Build history of the part. All positions in model axes, mm. Face numbers are marked on the shaded views. A direction names the side the tool comes from. Round coordinates to 2 decimals unless told otherwise and drop trailing zeros. Write each loop counter-clockwise with the first axis right and the second up, starting at its lowest first coordinate (ties: lowest second). Pieces come first, ordered by that corner, then holes. Notation, with made-up numbers: (60.5, 39.5) -> (81.5, 39.5) arc R25 ccw to (81.5, 66.5) -> close; hole circle Ø10 at (52, 14). An arc over 180 degrees is marked (long way). Return JSON: item names as keys, results as strings.
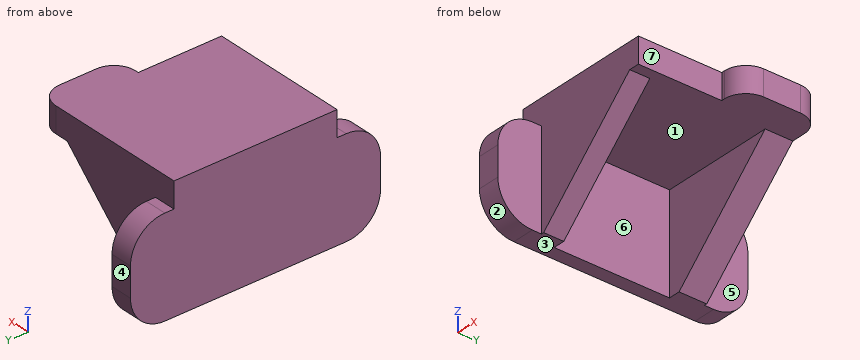
Autodesk Inventor part; units mm, degrees
ref_plane "YZ Plane" through (0, 0, 0) normal (1, 0, 0) x (0, 1, 0)
ref_plane "XZ Plane" through (0, 0, 0) normal (0, 1, 0) x (-1, 0, 0)
ref_plane "XY Plane" through (0, 0, 0) normal (0, 0, 1) x (1, 0, 0)
sketch "Sketch1" plane through (0, 0, 0) normal (0, 0, 1) x (1, 0, 0)
  line L0 (0, 0) -> (0, 60.76)
  line L1 (0, 60.76) -> (51.9, 60.76)
  line L2 (51.9, 31.06) -> (51.9, 0)
  line L3 (51.9, 0) -> (0, 0)
  line L4 (51.9, 60.76) -> (61.1, 60.76)
  line L5 (61.1, 60.76) -> (61.1, 31.06)
  line L6 (61.1, 31.06) -> (51.9, 31.06)
  dimension "d0" = 60.76
  dimension "d1" = 51.9
  dimension "d2" = 9.2
  dimension "d3" = 29.7
extrude "Extrusion1" add sketch "Sketch1" along normal blind 9.5
fillet "Fillet1" radius 8 2 edges at (61.1, 60.76, 4.75) (61.1, 31.06, 4.75)
sketch "Sketch2" plane through (0, 0, 0) normal (0, -1, 0) x (1, 0, 0)
  line L0 (51.9, 0) -> (0, 0)
  line L1 (0, -36.5) -> (0, 0)
  line L2 (0, -36.5) -> (9.3, -36.5)
  line L3 (9.3, -36.5) -> (48, 0)
  point P0 (0, 9.5)
  dimension "d7" = 46
  dimension "d8" = 3.9
  dimension "d9" = 9.3
extrude "Extrusion2" add sketch "Sketch2" against normal blind 7.5
sketch "Sketch3" plane through (0, 60.76, 9.5) normal (0, 1, 0) x (1, 0, 0)
  line L0 (0, 46) -> (0, 9.5)
  line L1 (48, 9.5) -> (0, 9.5)
  line L2 (48, 9.5) -> (9.3, 46)
  line L3 (9.3, 46) -> (0, 46)
extrude "Extrusion3" add sketch "Sketch3" against normal blind 10.3
sketch "Sketch4" plane through (0, 0, 9.5) normal (-1, 0, 0) x (0, 0, 1)
  line L0 (-46, 60.76) -> (0, 60.76)
  line L1 (-9.5, 7.5) -> (-9.5, 50.46)
  line L2 (-46, 0) -> (-46, 7.5)
  line L3 (-46, -16.2) -> (-46, 76.96)
  line L4 (-9.5, 76.96) -> (-9.5, -16.2)
  line L5 (-9.5, -16.2) -> (-46, -16.2)
  line L6 (-9.5, 76.96) -> (-46, 76.96)
  point P0 (-9.5, 0)
  dimension "d15" = 93.16
  dimension "d16" = 16.2
extrude "Extrusion4" add sketch "Sketch4" against normal blind 8.3
sketch "Sketch5" plane through (8.3, 0, 9.5) normal (1, 0, 0) x (0, 0, -1)
  line L0 (9.5, 50.46) -> (46, 50.46)
  line L1 (9.5, 7.5) -> (9.5, 50.46)
  line L2 (46, 7.5) -> (9.5, 7.5)
  line L3 (46, 7.5) -> (46, 50.46)
  point P0 (9.5, 0)
extrude "Extrusion5" cut sketch "Sketch5" against normal blind 3.3
fillet "Fillet2" radius 12.8 4 edges at (4.15, 76.96, -36.5) (4.15, -16.2, -36.5) (4.15, -16.2, 0) (4.15, 76.96, 0)
properties part number "FelixOriginalBase"
Q1. Saw through at D-D on y = 27.5. List the corners of the cut face in (x, z).
Verdict:
{"outline": "(0, -36.5) -> (5, -36.5) -> (5, 0) -> (51.9, 0) -> (51.9, 9.5) -> (0, 9.5) -> close"}
Q2. Pin check, flat tips, straight feed: pin 1 Ø1.7 at (x, y) = (6, 62) entering from +Z; pin 2 Ø5 at (x, z) = (42.5, -3) entering from -Y; pin 3 Ø8 at (x, z) = (34.5, 4) entering from +Y. Stop position of each tip, or through.
Verdict:
{"pin 1": "stops at z = 0", "pin 2": "stops at y = 0", "pin 3": "stops at y = 60.76"}
Q3. 3-axis set-ups, long thin cutter, end or side, ignore diameter. For the marked faces 4, 5, 6 and 7: which of +Z, -Z, +X, -X, +Y, -Y reach the whole face in a straight line?
Verdict:
{"face 4": "+Z, -Z, +X, -X, +Y", "face 5": "+Z, -Z, +X, +Y", "face 6": "-Z, +X", "face 7": "+Z, -Z, +X, -Y"}
Q4. Saw through at A-A on y = 6.5. List the corners of the cut face in (x, z), then the cut area to 3 significant figures.
Verdict:
{"outline": "(0, -36.5) -> (9.3, -36.5) -> (48, 0) -> (51.9, 0) -> (51.9, 9.5) -> (0, 9.5) -> close", "area": "1,540 mm²"}
Q5. Saw through at B-B on x = 36.5. List the corners of the cut face in (y, z), then the cut area to 3 significant figures.
Verdict:
{"outline": "(0, -10.85) -> (7.5, -10.85) -> (7.5, 0) -> (50.46, 0) -> (50.46, -10.85) -> (60.76, -10.85) -> (60.76, 9.5) -> (0, 9.5) -> close", "area": "770 mm²"}
Q6. Two-plate mould, pull along Y, no slides. Class the marked faces 1, 2 and 3: +Y half, -Y half, draft (parallel to the pull), parting line (faces both ways), or undercut.
Verdict:
{"face 1": "undercut", "face 2": "-Y half", "face 3": "draft"}
Q7. Saw through at C-C on z = -28.5. List the corners of the cut face in (x, y), then the cut area to 3 significant figures.
Verdict:
{"outline": "(0, -15.27) -> (8.3, -15.27) -> (8.3, 0) -> (17.78, 0) -> (17.78, 7.5) -> (5, 7.5) -> (5, 50.46) -> (17.78, 50.46) -> (17.78, 60.76) -> (8.3, 60.76) -> (8.3, 76.03) -> (0, 76.03) -> close", "area": "785 mm²"}
Q8. Wall check: L1, parallel to Y at x = 31, z = -2.5; L2, parallel to X at y = 55, z = 2; L3, parallel to X at y = 9, z = -22. Give the ranges that are in metal, low to high.
Verdict:
{"L1": "y = 0 to 7.5, 50.46 to 60.76", "L2": "x = 0 to 60.78", "L3": "x = 0 to 5"}
